from build123d import *

# Parameters (mm, degrees)
SKETCH_1_W          = 30
SKETCH_1_H          = 40
EXTRUDE_1_DEPTH     = 3
SKETCH_2_R          = 5.1
SKETCH_2_R_2        = 1.575
CUT_EXTRUDE_1_DEPTH = 51.089919145
FILLET_1_R          = 10
FILLET_2_R          = 4


with BuildPart() as part:
    # 草图1 → 凸台-拉伸1 (new body)
    with BuildSketch(Plane.XY):
        with Locations((15, -20)):
            Rectangle(SKETCH_1_W, SKETCH_1_H)
    extrude(amount=EXTRUDE_1_DEPTH)

    # 草图2 → 切除-拉伸1 (cut, through all)
    with BuildSketch(Plane.XY.offset(3)):
        with Locations((15, -12.5)):
            Circle(SKETCH_2_R)
        with Locations((5, -25)):
            Circle(SKETCH_2_R_2)
        with Locations(Location((5, -35, 0), (0, 0, 180))):
            Circle(SKETCH_2_R_2)
        with Locations((25, -35)):
            Circle(SKETCH_2_R_2)
        with Locations(Location((25, -25, 0), (0, 0, 180))):
            Circle(SKETCH_2_R_2)
    extrude(amount=-CUT_EXTRUDE_1_DEPTH, mode=Mode.SUBTRACT)

    # 圆角1
    fillet_1_edges = [part.edges().sort_by_distance(p)[0] for p in [
        (0, 0, 1.5),
        (30, 0, 1.5),
    ]]
    fillet(fillet_1_edges, radius=FILLET_1_R)

    # 圆角2
    fillet_2_edges = [part.edges().sort_by_distance(p)[0] for p in [
        (30, -40, 1.5),
        (0, -40, 1.5),
    ]]
    fillet(fillet_2_edges, radius=FILLET_2_R)


solid = part.part
Source: CAD feature listing. Evaluate the final solid. Frame: model axes, mm. Coordinates: 2 decimals unless noted, no trailing zeros. Loops run counter-clockwise (first coordinate to the right, second up) from the corner with the lowest first, then second, coordinate; pieces in that order, holes last. Notation, with made-up numbers: (66.5, 66) -> (109.5, 66) arc R9 cw to (109.5, 76) -> close; hole circle Ø11 at (18, 66.5). An arc over 180 degrees is marked (long way). Answer in a Markdown table with one row per item. Add a question column.
Q1. Section A-A on x = 15. Return the cut outline in (y, z), and give its area (3 significant figures).
Q2. Section C-C on y = -25. Return the cut outline in (x, z) (3 decimals), and give its area (3 significant figures).
Q3. Pull-direction query (Y, two-part tool) for faces 1 (the face through (28.797, -38.859, 1.521)), 2 (the face through (19.864, -10.968, 1.521)), 3 (the face through (15, -20, 0)), 4 (the face through (15, 0, 1)); classes: pulls with the +Y half, pulls with the -Y half, needs draft (parallel to the pull), parting line crosses it, or undercut.
Q4. Section B-B on z = 2.1. Return the cut outline in (x, y) (3 decimals).
Q5. Ray query, line 1 along Y through (x, z) = (15, 2); line 2 along X through (y, z) = (-13.5, 2.45); line 3 along Y through (x, z) = (25, 1.25) (3 decimals). Return the intervals inside material, ascending.
Q6. Section D-D on x = 6. Return the cut outline in (y, z), and give its area (3 significant figures).
Computed values:
| question | item | result |
|---|---|---|
| 1 | outline | (-40, 0) -> (-17.6, 0) -> (-17.6, 3) -> (-40, 3) -> close; (-7.4, 0) -> (0, 0) -> (0, 3) -> (-7.4, 3) -> close |
| 1 | area | 89.4 mm^2 |
| 2 | outline | (0, 0) -> (3.425, 0) -> (3.425, 3) -> (0, 3) -> close; (6.575, 0) -> (23.425, 0) -> (23.425, 3) -> (6.575, 3) -> close; (26.575, 0) -> (30, 0) -> (30, 3) -> (26.575, 3) -> close |
| 2 | area | 71.1 mm^2 |
| 3 | face 1 | pulls with the -Y half |
| 3 | face 2 | undercut |
| 3 | face 3 | needs draft |
| 3 | face 4 | pulls with the +Y half |
| 4 | outline | (0, -36) arc R4 ccw to (4, -40) -> (26, -40) arc R4 ccw to (30, -36) -> (30, -10) arc R10 ccw to (20, 0) -> (10, 0) arc R10 ccw to (0, -10) -> close; hole circle Ø3.15 at (5, -35); hole circle Ø3.15 at (5, -25); hole circle Ø10.2 at (15, -12.5); hole circle Ø3.15 at (25, -35); hole circle Ø3.15 at (25, -25) |
| 5 | line 1 | y = -40 to -17.6, -7.4 to 0 |
| 5 | line 2 | x = 0 to 10, 20 to 30 |
| 5 | line 3 | y = -40 to -36.575, -33.425 to -26.575, -23.425 to -1.34 |
| 6 | outline | (-40, 0) -> (-36.22, 0) -> (-36.22, 3) -> (-40, 3) -> close; (-33.78, 0) -> (-26.22, 0) -> (-26.22, 3) -> (-33.78, 3) -> close; (-23.78, 0) -> (-0.83, 0) -> (-0.83, 3) -> (-23.78, 3) -> close |
| 6 | area | 103 mm^2 |
